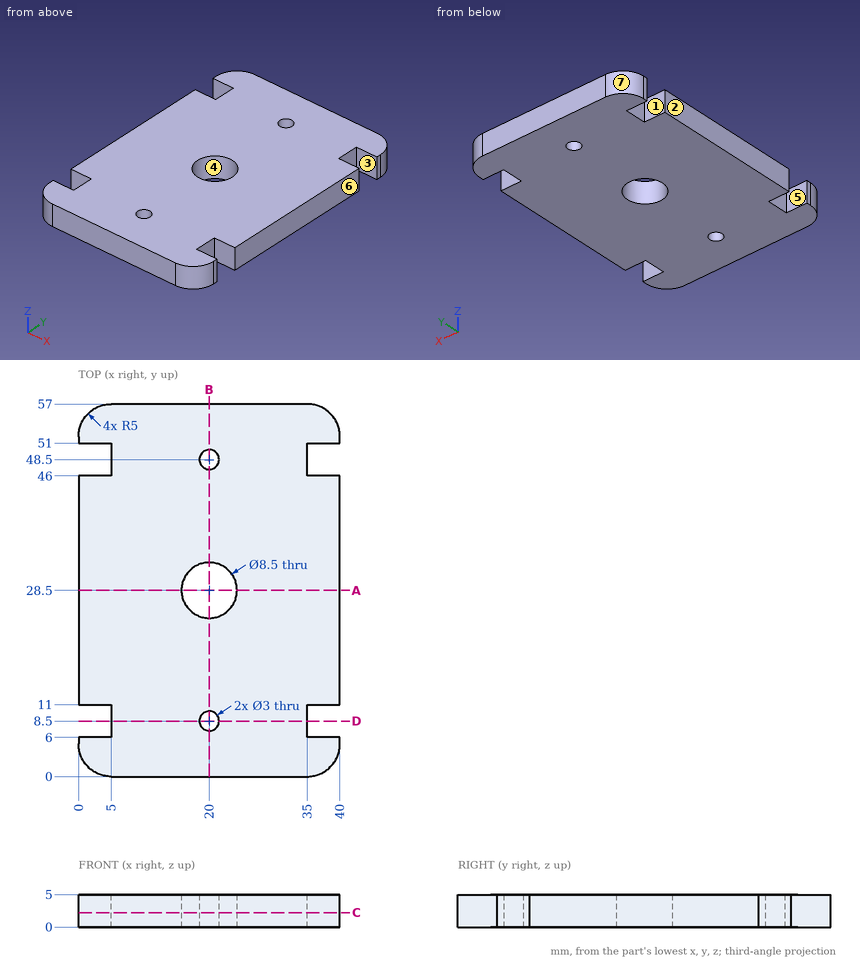
Study the drawing (mm; zero at the part's minimum x, y, z) and answer. A direction names the side the tool comes from. Round coordinates to 2 decimals unless told otherwise and drop trailing zeros. Write each loop counter-clockwise with the first axis right and the second up, starting at its lowest first coordinate (ties: lowest second). Pieces come first, ordered by that corner, then holes. Notation, with made-up numbers: (-38, 84.25) -> (13, 84.25) arc R21 ccw to (13, 101.25) -> close; hole circle Ø7 at (25, -34). An arc over 180 degrees is marked (long way). Write item = value, one per line.
1) Section C-C on z = 2.25 is taken. Write down the section's boundary in (x, y).
Check values:
outline = (0, 5) arc R5 ccw to (5, 0) -> (35, 0) arc R5 ccw to (40, 5) -> (40, 6) -> (35, 6) -> (35, 11) -> (40, 11) -> (40, 46) -> (35, 46) -> (35, 51) -> (40, 51) -> (40, 52) arc R5 ccw to (35, 57) -> (5, 57) arc R5 ccw to (0, 52) -> (0, 51) -> (5, 51) -> (5, 46) -> (0, 46) -> (0, 11) -> (5, 11) -> (5, 6) -> (0, 6) -> close; hole circle Ø8.5 at (20, 28.5); hole circle Ø3 at (20, 8.5); hole circle Ø3 at (20, 48.5)
2) Given pin 1 (1.5 mm diameter, centred on y = 49, z = 3.5, fed in from +X); pin 2 (1.5 mm diameter, centred on x = 36.5, z = 3, fed in from -Y); pin 3 (2.5 mm diameter, centred on x = 3, z = 1.5, fed in from +Y), each flat-ended and moving along its own axis, determine where each tip first touches the part or whether it passes through.
Check values:
pin_1 = 35
pin_2 = 0.06
pin_3 = 56.94
3) Section D-D on y = 8.5 is taken. Write down the section's boundary in (x, z).
Check values:
outline = (5, 0) -> (18.5, 0) -> (18.5, 5) -> (5, 5) -> close; (21.5, 0) -> (35, 0) -> (35, 5) -> (21.5, 5) -> close
4) For a pull along X with two mould halves and no side action, classify the marked faces 4, 5, 6 and 7 as released by +X, released by -X, zero draft, split by the parting line, or undercut.
Check values:
face_4 = undercut
face_5 = zero draft
face_6 = released by +X
face_7 = released by -X
5) Which of the six approach directions +Z, -Z, +X, -X, +Y, -Y give full straight-line access (tool end or side, diameter ignored) to the marked faces 1, 2 and 3?
Check values:
face_1 = +Z, -Z, -X
face_2 = +Z, -Z, -X, +Y, -Y
face_3 = +Z, -Z, +X
6) Section B-B on x = 20 is taken. Write down the section's boundary in (y, z), plus the area to 4 significant figures.
Check values:
outline = (0, 0) -> (7, 0) -> (7, 5) -> (0, 5) -> close; (10, 0) -> (24.25, 0) -> (24.25, 5) -> (10, 5) -> close; (32.75, 0) -> (47, 0) -> (47, 5) -> (32.75, 5) -> close; (50, 0) -> (57, 0) -> (57, 5) -> (50, 5) -> close
area = 212.5 mm²
7) Section A-A on y = 28.5 is taken. Write down the section's boundary in (x, z).
Check values:
outline = (0, 0) -> (15.75, 0) -> (15.75, 5) -> (0, 5) -> close; (24.25, 0) -> (40, 0) -> (40, 5) -> (24.25, 5) -> close
8) Straight lines are drawn through the part: line 1 along Y through (x, z) = (20, 2.5); line 2 along Y through (x, z) = (37.5, 2.4); line 3 along Y through (x, z) = (4, 2.35). For each, find the intervals that lie inside material, in ascending order. Write a range as [from, to].
Check values:
line_1 = [0, 7], [10, 24.25], [32.75, 47], [50, 57]
line_2 = [0.67, 6], [11, 46], [51, 56.33]
line_3 = [0.1, 6], [11, 46], [51, 56.9]
